from build123d import *

# Parameters (mm, degrees)
SKETCH2_R           = 105
SKETCH2_R_2         = 65
BOSS_EXTRUDE1_START = -50
SKETCH4_W           = 360
SKETCH4_H           = 360
SKETCH4_R           = 105
BOSS_EXTRUDE1_DEPTH = 50
FILLET1_R           = 20
SKETCH5_R           = 105
BOSS_EXTRUDE2_DEPTH = 50
SKETCH6_R           = 30
CUT_EXTRUDE1_DEPTH  = 10
CUT_EXTRUDE2_REACH  = 848.699
SKETCH7_R           = 15
CIRPATTERN1_COUNT   = 4
SKETCH8_R           = 30
CUT_EXTRUDE4_DEPTH  = 10
CUT_EXTRUDE5_REACH  = 734.735
SKETCH10_R          = 15
CIRPATTERN2_COUNT   = 4
CHAMFER1_SIZE       = 10


with BuildPart() as part:
    # Sweep-Thin1: sweep along a path in Sketch1
    with BuildLine(Plane.XY) as sweep_thin1_path:
        Line((0, 0), (-150, 0))
        ThreePointArc((-150, 0), (-333.847763109, 76.152236891), (-410, 260))
        Line((-410, 260), (-410, 410))
    # Sketch2 → Sweep-Thin1 (sweep)
    with BuildSketch(Plane(origin=(0, 0, 0), x_dir=(0, 0, -1), z_dir=(1, 0, 0))):
        Circle(SKETCH2_R)
        Circle(SKETCH2_R_2, mode=Mode.SUBTRACT)
    sweep(path=sweep_thin1_path.line)

    # Sketch4 → Boss-Extrude1 (add)
    with BuildSketch(Plane(origin=(0, 0, 0), x_dir=(0, 0, -1), z_dir=(1, 0, 0)).offset(BOSS_EXTRUDE1_START)):
        Rectangle(SKETCH4_W, SKETCH4_H)
        with Locations(Location((0, 0, 0), (0, 0, 270))):
            Circle(SKETCH4_R, mode=Mode.SUBTRACT)
    extrude(amount=BOSS_EXTRUDE1_DEPTH)

    # Fillet1
    fillet1_edges = [part.edges().sort_by_distance(p)[0] for p in [
        (-25, 180, -180),
        (-25, -180, -180),
        (-25, -180, 180),
        (-25, 180, 180),
    ]]
    fillet(fillet1_edges, radius=FILLET1_R)

    # Sketch5 → Boss-Extrude2 (add)
    with BuildSketch(Plane(origin=(0, 410, 0), x_dir=(1, 0, 0), z_dir=(0, 1, 0))):
        with BuildLine():
            Line((-570, -180), (-250, -180))
            ThreePointArc((-250, -180), (-235.857864376, -174.142135624), (-230, -160))
            Line((-230, -160), (-230, 160))
            ThreePointArc((-230, 160), (-235.857864376, 174.142135624), (-250, 180))
            Line((-250, 180), (-570, 180))
            ThreePointArc((-570, 180), (-584.142135624, 174.142135624), (-590, 160))
            Line((-590, 160), (-590, -160))
            ThreePointArc((-590, -160), (-584.142135624, -174.142135624), (-570, -180))
        make_face()
        with Locations(Location((-410, 0, 0), (0, 0, 180))):
            Circle(SKETCH5_R, mode=Mode.SUBTRACT)
    extrude(amount=-BOSS_EXTRUDE2_DEPTH)

    # Sketch6 → Cut-Extrude1 (cut)
    with BuildSketch(Plane(origin=(0, 410, 0), x_dir=(1, 0, 0), z_dir=(0, 1, 0))):
        with Locations(Location((-540, 130, 0), (0, 0, 180))):
            Circle(SKETCH6_R)
    cut_extrude1 = extrude(amount=-CUT_EXTRUDE1_DEPTH, mode=Mode.SUBTRACT)

    # Sketch7 → Cut-Extrude2 (cut, up to next)
    with BuildSketch(Plane(origin=(0, 400, 0), x_dir=(1, 0, 0), z_dir=(0, 1, 0)), mode=Mode.PRIVATE) as cut_extrude2_sk1:
        with Locations(Location((-540, 130, 0), (0, 0, 180))):
            Circle(SKETCH7_R)
    cut_extrude2_tool1 = extrude(cut_extrude2_sk1.sketch, amount=-CUT_EXTRUDE2_REACH, mode=Mode.PRIVATE) & part.part
    cut_extrude2 = cut_extrude2_tool1.solids().sort_by_distance((-540, 400, -130))[0]
    add(cut_extrude2, mode=Mode.SUBTRACT)

    # CirPattern1: Cut-Extrude1, Cut-Extrude2 ×4 about axis
    cirpattern1_axis = Axis((-410, 0, 0), (0, 1, 0))
    add([cut_extrude1.rotate(cirpattern1_axis, i * 360 / CIRPATTERN1_COUNT) for i in range(1, CIRPATTERN1_COUNT)], mode=Mode.SUBTRACT)
    add([cut_extrude2.rotate(cirpattern1_axis, i * 360 / CIRPATTERN1_COUNT) for i in range(1, CIRPATTERN1_COUNT)], mode=Mode.SUBTRACT)

    # Sketch8 → Cut-Extrude4 (cut)
    with BuildSketch(Plane(origin=(0, 0, 0), x_dir=(0, 0, -1), z_dir=(1, 0, 0))):
        with Locations((-130, 130)):
            Circle(SKETCH8_R)
    cut_extrude4 = extrude(amount=-CUT_EXTRUDE4_DEPTH, mode=Mode.SUBTRACT)

    # Sketch10 → Cut-Extrude5 (cut, up to next)
    with BuildSketch(Plane(origin=(-10, 0, 0), x_dir=(0, 0, -1), z_dir=(1, 0, 0)), mode=Mode.PRIVATE) as cut_extrude5_sk1:
        with Locations((-130, 130)):
            Circle(SKETCH10_R)
    cut_extrude5_tool1 = extrude(cut_extrude5_sk1.sketch, amount=-CUT_EXTRUDE5_REACH, mode=Mode.PRIVATE) & part.part
    cut_extrude5 = cut_extrude5_tool1.solids().sort_by_distance((-10, 130, 130))[0]
    add(cut_extrude5, mode=Mode.SUBTRACT)

    # CirPattern2: Cut-Extrude4, Cut-Extrude5 ×4 about axis
    cirpattern2_axis = Axis((0, 0, 0), (1, 0, 0))
    add([cut_extrude4.rotate(cirpattern2_axis, i * 360 / CIRPATTERN2_COUNT) for i in range(1, CIRPATTERN2_COUNT)], mode=Mode.SUBTRACT)
    add([cut_extrude5.rotate(cirpattern2_axis, i * 360 / CIRPATTERN2_COUNT) for i in range(1, CIRPATTERN2_COUNT)], mode=Mode.SUBTRACT)

    # Chamfer1
    chamfer1_edges = [part.edges().sort_by_distance(p)[0] for p in [
        (0, 0, 65),
        (-410, 410, 65),
    ]]
    chamfer(chamfer1_edges, length=CHAMFER1_SIZE)


solid = part.part
Check sheet for the modelled part. Datum: model origin and axes. Units: mm. A direction names the side the tool comes from. Round coordinates to 2 decimals unless told otherwise and drop trailing zeros. Loops run counter-clockwise (first coordinate to the right, second up) from the corner with the lowest first, then second, coordinate; pieces in that order, holes last. Notation, with made-up numbers: M -18.5,19 L 2.5,19 A23 ccw 2.5,31 Z; hole C 12,5.5 d11. An arc over 180 degrees is marked long. One line per item, written item: value.
(1) Sectioned sample at A-A, the plane z = 0. Record the cut outline in (x, y), then the cut area to 3 significant figures.
Computed values:
outline: M -590,360 L -515,360 L -515,260 A365 ccw -150,-105 L -50,-105 L -50,-180 L 0,-180 L 0,-75 L -10,-65 L -150,-65 A325 cw -475,260 L -475,400 L -485,410 L -590,410 Z; M -345,260 A195 ccw -150,65 L -10,65 L 0,75 L 0,180 L -50,180 L -50,105 L -150,105 A155 cw -305,260 L -305,360 L -230,360 L -230,410 L -335,410 L -345,400 Z
area: 71,500 mm^2
(2) Thickness scan on line 1 (X direction, y = 388.5, z = -130); line 2 (Z direction, x = -33, y = -130); line 3 (X direction, y = 352.5, z = 0). Record the ranges inside material, lowest first.
Computed values:
line 1: x = -590 to -555, -525 to -295, -265 to -230
line 2: z = -180 to -145, -115 to 115, 145 to 180
line 3: x = -515 to -475, -345 to -305
(3) Sectioned sample at B-B, the plane x = -540. Record the cut outline in (y, z), then the cut area to 3 significant figures.
Computed values:
outline: M 360,-180 L 410,-180 L 410,-160 L 400,-160 L 400,-145 L 360,-145 Z; M 360,-115 L 400,-115 L 400,-100 L 410,-100 L 410,100 L 400,100 L 400,115 L 360,115 Z; M 360,145 L 400,145 L 400,160 L 410,160 L 410,180 L 360,180 Z
area: 14,400 mm^2
(4) Depth check by flat-ended pin: pin 1 Ø10 at (y, z) = (43.5, 134) entering from -X; pin 2 Ø25 at (x, z) = (-18.5, -3) entering from +Y; pin 3 Ø3 at (y, z) = (121, -86.5) entering from -X. Enter the tip coordinate at first touch or a pass-through.
Computed values:
pin 1: stops at x = -50
pin 2: stops at y = 180
pin 3: stops at x = -440.17
(5) Access from +Z, -Z, +X, -X, +Y, -Y to the whole of each face (thin tool, end or side, straight path). Record for faces 4 (the face through (-4.93, 152.111, -150.275)), 5 (the face through (-281.953, 380.28, 115.128)), 6 (the face through (-510.255, 405.07, 126.095)).
Computed values:
face 4: +X
face 5: +Y, -Y
face 6: +Y
(6) Sectioned sample at C-C, the plane y = 130. Count the separate pieces of the cut face and the enclosed holes in it, then the cut area to 3 significant figures.
Computed values:
separate pieces: 4
enclosed holes: 1
area: 40,500 mm^2
(7) Release check for a two-part mould opening along Z. For faces 1 (the face through (-100.7, -31.54, -100.15)), 2 (the face through (-10, 144, 124)), 3 (the face through (-236.014, 385.35, 174.297)) record: +Z half, -Z half, draft (parallel to the pull), parting line (faces both ways), or undercut.
Computed values:
face 1: parting line
face 2: undercut
face 3: +Z half
